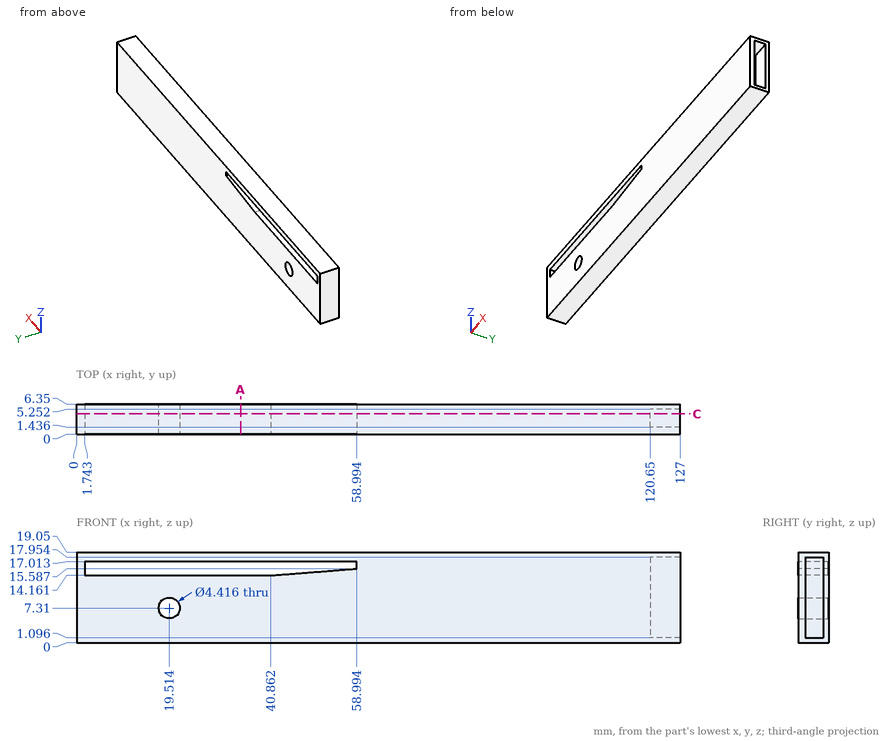
Source: three-view drawing plus pictorial views. Frame: mm from the lowest corner of the part. Round coordinates to 2 decimals unless told otherwise and drop trailing zeros. Loops run counter-clockwise (first coordinate to the right, second up) from the corner with the lowest first, then second, coordinate; pieces in that order, holes last.
Q1. First-contact query: P1, Ø1.5, axis at y = 3.5, z = 9, coming from the +X side; P2, Ø1.1, axis at y = 3, z = 16, coming from the -X side. Flat tips, straight axial feed; report the tip coordinate or a pass-through.
Q2. Section C-C, the plane y = 4.25. Return loops of the section in (x, z).
Q3. Ray query, line 1 (Z direction, x = 10, y = 4.25); line 2 (X direction, y = 2.25, z = 16); line 3 (X direction, y = 5, z = 10). Return the intervals inside material, ascending.
Q4. Section A-A, the plane x = 34.5. Return loops of the section in (y, z).
Solutions:
1. P1: stops at x = 120.65
1. P2: stops at x = 0
2. outline: (0, 0) - (127, 0) - (127, 1.1) - (120.65, 1.1) - (120.65, 17.95) - (127, 17.95) - (127, 19.05) - (0, 19.05) - close; hole (1.74, 14.16) - (40.86, 14.16) - (58.99, 15.59) - (58.99, 17.01) - (1.74, 17.01) - close; hole circle Ø4.42 at (19.51, 7.31)
3. line 1: z = 0 to 14.16, 17.01 to 19.05
3. line 2: x = 0 to 1.74, 58.99 to 120.65
3. line 3: x = 0 to 120.65
4. outline: (0, 0) - (6.35, 0) - (6.35, 14.16) - (0, 14.16) - close; (0, 17.01) - (6.35, 17.01) - (6.35, 19.05) - (0, 19.05) - close
